from build123d import *

# Parameters (mm, degrees)
EXTRUDE_2_DEPTH          = 5
EXTRUDE_3_DEPTH          = 27.5
FILLET_1_R               = 3.5
SKETCH_4_R               = 5
CUT_EXTRUDE_1_DEPTH      = 5
CUT_EXTRUDE_2_DEPTH      = 66.80653463
CUT_EXTRUDE_2_DEPTH_BACK = 1.5
SKETCH_6_R               = 2.5
CUT_EXTRUDE_3_DEPTH      = 10


with BuildPart() as part:
    # ｽｹｯﾁ1 → ﾎﾞｽ - 押し出し2 (new body)
    with BuildSketch(Plane(origin=(0, 0, 0), x_dir=(1, 0, 0), z_dir=(0, 1, 0))):
        with BuildLine():
            Line((-58, -14.5), (-58, 14.5))
            Line((-58, 14.5), (-55.2, 14.5))
            ThreePointArc((-55.2, 14.5), (-53.785786438, 13.914213562), (-53.2, 12.5))
            Line((-53.2, 12.5), (-53.2, 10.9))
            Line((-53.2, 10.9), (-48.4, 10.9))
            Line((-48.4, 10.9), (-48.4, 12.5))
            ThreePointArc((-48.4, 12.5), (-47.814213562, 13.914213562), (-46.4, 14.5))
            Line((-46.4, 14.5), (-40.7, 14.5))
            ThreePointArc((-40.7, 14.5), (-39.285786438, 13.914213562), (-38.7, 12.5))
            Line((-38.7, 12.5), (-38.7, 10.9))
            Line((-38.7, 10.9), (38.7, 10.9))
            Line((38.7, 10.9), (38.7, 12.5))
            ThreePointArc((38.7, 12.5), (39.285786438, 13.914213562), (40.7, 14.5))
            Line((40.7, 14.5), (46.4, 14.5))
            ThreePointArc((46.4, 14.5), (47.814213562, 13.914213562), (48.4, 12.5))
            Line((48.4, 12.5), (48.4, 10.9))
            Line((48.4, 10.9), (53.2, 10.9))
            Line((53.2, 10.9), (53.2, 12.5))
            ThreePointArc((53.2, 12.5), (53.785786438, 13.914213562), (55.2, 14.5))
            Line((55.2, 14.5), (58, 14.5))
            Line((58, 14.5), (58, -14.5))
            Line((58, -14.5), (55.2, -14.5))
            ThreePointArc((55.2, -14.5), (53.785786438, -13.914213562), (53.2, -12.5))
            Line((53.2, -12.5), (53.2, -10.9))
            Line((53.2, -10.9), (48.4, -10.9))
            Line((48.4, -10.9), (48.4, -12.5))
            ThreePointArc((48.4, -12.5), (47.814213562, -13.914213562), (46.4, -14.5))
            Line((46.4, -14.5), (40.7, -14.5))
            ThreePointArc((40.7, -14.5), (39.285786438, -13.914213562), (38.7, -12.5))
            Line((38.7, -12.5), (38.7, -10.9))
            Line((38.7, -10.9), (-38.7, -10.9))
            Line((-38.7, -10.9), (-38.7, -12.5))
            ThreePointArc((-38.7, -12.5), (-39.285786438, -13.914213562), (-40.7, -14.5))
            Line((-40.7, -14.5), (-46.4, -14.5))
            ThreePointArc((-46.4, -14.5), (-47.814213562, -13.914213562), (-48.4, -12.5))
            Line((-48.4, -12.5), (-48.4, -10.9))
            Line((-48.4, -10.9), (-53.2, -10.9))
            Line((-53.2, -10.9), (-53.2, -12.5))
            ThreePointArc((-53.2, -12.5), (-53.785786438, -13.914213562), (-55.2, -14.5))
            Line((-55.2, -14.5), (-58, -14.5))
        make_face()
    extrude(amount=EXTRUDE_2_DEPTH)

    # ｽｹｯﾁ3 → ﾎﾞｽ - 押し出し3 (add)
    with BuildSketch(Plane(origin=(0, 5, 0), x_dir=(1, 0, 0), z_dir=(0, 1, 0))):
        with BuildLine():
            Line((-44.9, 10.9), (44.9, 10.9))
            ThreePointArc((44.9, 10.9), (47.374873734, 9.874873734), (48.4, 7.4))
            Line((48.4, 7.4), (48.4, -7.4))
            ThreePointArc((48.4, -7.4), (47.374873734, -9.874873734), (44.9, -10.9))
            Line((44.9, -10.9), (-44.9, -10.9))
            ThreePointArc((-44.9, -10.9), (-47.374873734, -9.874873734), (-48.4, -7.4))
            Line((-48.4, -7.4), (-48.4, 7.4))
            ThreePointArc((-48.4, 7.4), (-47.374873734, 9.874873734), (-44.9, 10.9))
        make_face()
    extrude(amount=EXTRUDE_3_DEPTH)

    # ﾌｨﾚｯﾄ1
    fillet_1_edges = [part.edges().sort_by_distance(p)[0] for p in [
        (47.374873734, 32.5, -9.874873734),
        (0, 32.5, -10.9),
        (-47.374873734, 32.5, -9.874873734),
        (-48.4, 32.5, 0),
        (-47.374873734, 32.5, 9.874873734),
        (0, 32.5, 10.9),
        (47.374873734, 32.5, 9.874873734),
        (48.4, 32.5, 0),
    ]]
    fillet(fillet_1_edges, radius=FILLET_1_R)

    # ｽｹｯﾁ4 → ｶｯﾄ - 押し出し1 (cut)
    with BuildSketch(Plane.ZY.offset(48.4)):
        with Locations((0, 15)):
            Circle(SKETCH_4_R)
    cut_extrude_1 = extrude(amount=-CUT_EXTRUDE_1_DEPTH, mode=Mode.SUBTRACT)

    # ﾐﾗｰ1: ｶｯﾄ - 押し出し1 across plane
    add(cut_extrude_1.mirror(Plane(origin=(0, 0, 0), x_dir=(0, 0, 1), z_dir=(1, 0, 0))), mode=Mode.SUBTRACT)

    # ｽｹｯﾁ5 → ｶｯﾄ - 押し出し2 (cut, two sides: drawn at the far end of the back side and taken through both)
    with BuildSketch(Plane(origin=(0, 5, 0), x_dir=(1, 0, 0), z_dir=(0, 1, 0)).offset(-CUT_EXTRUDE_2_DEPTH_BACK)):
        with BuildLine():
            Line((-53.2, -4.6), (-58, -4.6))
            Line((-58, -4.6), (-58, 4.6))
            Line((-58, 4.6), (-53.2, 4.6))
            ThreePointArc((-53.2, 4.6), (-48.6, 0), (-53.2, -4.6))
        make_face()
        with BuildLine():
            Line((58, -4.6), (58, 4.6))
            Line((58, 4.6), (53.2, 4.6))
            ThreePointArc((53.2, 4.6), (48.6, 0), (53.2, -4.6))
            Line((53.2, -4.6), (58, -4.6))
        make_face()
    extrude(amount=CUT_EXTRUDE_2_DEPTH + CUT_EXTRUDE_2_DEPTH_BACK, mode=Mode.SUBTRACT)

    # ｽｹｯﾁ6 → ｶｯﾄ - 押し出し3 (cut)
    with BuildSketch(Plane(origin=(0, 3.5, 0), x_dir=(1, 0, 0), z_dir=(0, 1, 0))):
        with Locations(Location((-54, 0, 0), (0, 0, 270))):
            Circle(SKETCH_6_R)
        with Locations(Location((54, 0, 0), (0, 0, 270))):
            Circle(SKETCH_6_R)
    extrude(amount=-CUT_EXTRUDE_3_DEPTH, mode=Mode.SUBTRACT)


solid = part.part
Read the model definition and answer for the solid it produces. Units are mm, in the model's axes. A direction names the side the tool comes from. Round coordinates to 2 decimals unless told otherwise and drop trailing zeros. Loops run counter-clockwise (first coordinate to the right, second up) from the corner with the lowest first, then second, coordinate; pieces in that order, holes last.
Q1. Each of these flat-tipped pins is pushed along its axis until it touches: pin 1 (9 mm diameter, centred on y = 15, z = 0, fed in from +X); pin 2 (1 mm diameter, centred on y = 9.5, z = -7, fed in from -X); pin 3 (4 mm diameter, centred on x = -2, y = 8, fed in from -Z). Where does it stop, or does it pass through?
Q2. Section A-A on z = 0 is taken. Give the number of separate pieces and of enclosed holes in the cut face, and give its area (3 significant figures).
Q3. Consider probe 1 along X at (y, z) = (1.05, 0); probe 2 along Z at (x, y) = (-40, 18.5); probe 3 along Y at (x, z) = (48, -0.75). Determine where each line is inside the solid, lowest interval first.
Q4. Determine the mould class of faces 5 (the face through (51.56, 1.77, -0.54)), 6 (the face through (43.4, 15, 0)), 7 (the face through (-44, 2, 14.5)) for opening direction X: released by +X, released by -X, zero draft, split by the parting line, or undercut.
Q5. Which of the six approach directions +Z, -Z, +X, -X, +Y, -Y give full straight-line access (tool end or side, diameter ignored) to faces 1 (the face through (-48.4, 19.5, 3.4)), 2 (the face through (51, 2, 10.9)), 3 (the face through (53.77, 2.46, -13.9)), 4 (the face through (-48.6, 4.2, -0.1))?
Q6. Section B-B on y = 15 is taken. Write down the section's boundary in (x, z).
Q7. Section C-C on x = -22 is taken. Write down the section's boundary in (y, z).
Output:
1. pin 1: stops at x = 43.4
1. pin 2: stops at x = -48.4
1. pin 3: stops at z = -10.9
2. separate pieces: 3
2. enclosed holes: 0
2. area: 3,070 mm2
3. probe 1: x = -58 to -56.5, -51.5 to 51.5, 56.5 to 58
3. probe 2: z = -10.9 to 10.9
3. probe 3: y = 0 to 10.06, 19.94 to 30.62
4. face 5: undercut
4. face 6: released by +X
4. face 7: zero draft
5. face 1: +Z, -Z, -X, +Y
5. face 2: +Z, +Y, -Y
5. face 3: -Z, +Y, -Y
5. face 4: -X, +Y
6. outline: (-48.4, -7.4) arc R3.5 ccw to (-44.9, -10.9) - (44.9, -10.9) arc R3.5 ccw to (48.4, -7.4) - (48.4, -5) - (43.4, -5) - (43.4, 5) - (48.4, 5) - (48.4, 7.4) arc R3.5 ccw to (44.9, 10.9) - (-44.9, 10.9) arc R3.5 ccw to (-48.4, 7.4) - (-48.4, 5) - (-43.4, 5) - (-43.4, -5) - (-48.4, -5) - close
7. outline: (0, -10.9) - (29, -10.9) arc R3.5 ccw to (32.5, -7.4) - (32.5, 7.4) arc R3.5 ccw to (29, 10.9) - (0, 10.9) - close
